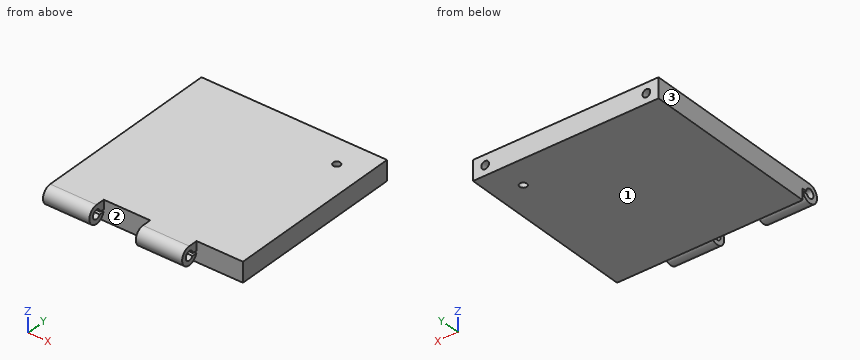
Autodesk Inventor part; units mm, degrees
ref_plane "YZ Plane" through (0, 0, 0) normal (1, 0, 0) x (0, 1, 0)
ref_plane "XZ Plane" through (0, 0, 0) normal (0, 1, 0) x (-1, 0, 0)
ref_plane "XY Plane" through (0, 0, 0) normal (0, 0, 1) x (1, 0, 0)
sketch "Sketch1" plane through (0, 0, 0) normal (0, 0, 1) x (1, 0, 0)
  line L0 (0, 0) -> (102.3, 0)
  line L1 (102.3, 0) -> (102.3, 100)
  line L2 (102.3, 100) -> (0, 100)
  line L3 (0, 100) -> (0, 0)
  dimension "d0" = 102.3
  dimension "d1" = 100
extrude "Extrusion1" add sketch "Sketch1" along normal blind 5
sketch "Sketch3" plane through (0, 0, 0) normal (-1, 0, 0) x (0, 0, 1)
  line L0 (5, 0) -> (0, 0)
  line L1 (0, 0) -> (0, -5)
  line L2 (0, -5) -> (5, -5)
  line L3 (5, -5) -> (5, 0)
  circle A0 centre (0, -5) radius 5
  circle A1 centre (0, -5) radius 2.5
  line L4 (-1.25, -2.8349) -> (-1.25, -0.1588)
  point P0 (0, 0)
  point P1 (0, -2.5)
  dimension "d15" = 5
  dimension "d16" = 5
  dimension "d17" = 5
  dimension "d18" = 2.5
  dimension "d19" = 1.25
extrude "Extrusion3" add sketch "Sketch3" against normal blind 25.575 contours L3 A0 L0 | A0 L2 A1 L1 | A0 L4 A1 L2
pattern_linear "Rectangular Pattern2" count 2 spacing 51.15 along (1, 0, 0) of "Extrusion3"
sketch "Sketch4" plane through (0, 0, 0) normal (0, 0, -1) x (-1, 0, 0)
  point P0 (0, 0)
sketch "Sketch5" plane through (0, 0, 0) normal (0, 0, -1) x (-1, 0, 0)
  line L0 (-102.3, 0) -> (-102.3, 100)
  line L1 (0, 0) -> (-102.3, 0)
  line L2 (-102.3, 0) -> (-102.3, 100)
  line L3 (-102.3, 100) -> (0, 100)
  line L4 (0, 100) -> (0, 0)
extrude "Extrusion4" add sketch "Sketch5" along normal blind 6
sketch "Sketch6" plane through (0, 0, 5) normal (0, 0, 1) x (1, 0, 0)
  line L0 (102.3, 100) -> (0, 100) construction
  line L1 (87.3, 100) -> (87.3, 84) construction
  line L2 (102.3, 0) -> (102.3, 100) construction
  point P0 (0, 0)
  dimension "d27" = 15
  dimension "d28" = 16
hole "Hole1" at (87.3, 84, 5) direction (0, 0, -1) diameter 4 end through all
sketch "Sketch8" plane through (51.15, -5, 5) normal (-1, 0, 0) x (0, 0, 1)
  point P0 (-5, 5)
sketch "Sketch9" plane through (0, 0, 5) normal (0, 0, 1) x (1, 0, 0)
  circle A0 centre (87.3, 84) radius 2 construction
  line L0 (87.3, 84) -> (102.3, 84) construction
  line L1 (102.3, 0) -> (102.3, 100) construction
  line L2 (87.3, 84) -> (87.3, 100) construction
  line L3 (76.725, 0) -> (102.3, 0)
  line L4 (102.3, 100) -> (0, 100)
  point P0 (0, 0)
  dimension "d45" = 15
  dimension "d46" = 16
  dimension "d57" = 100
sketch "Sketch10" plane through (0, 100, 5) normal (0, 1, 0) x (1, 0, 0)
  line L0 (0, 10) -> (0, 0) construction
  line L1 (0, 5.5) -> (102.7523, 5.5) construction
  line L2 (0, 11) -> (102.3, 11) construction
  point P0 (95.6, 5.5)
  point P1 (6.7, 5.5)
  point P2 (0, 6.25)
  dimension "d47" = 88.9
  dimension "d48" = 5.5
  dimension "d49" = 6.7
hole "Hole3" at (6.7, 100, -0.5) at (95.6, 100, -0.5) direction (0, -1, 0) diameter 4.25 depth 8 tip angle 118
properties part number "Hinge2"
The model under review builds one solid part; all positions refer to its coordinate system, in mm. Face numbers are marked on the shaded views. Give positions to 0.01 mm unless a question says otherwise; leave off trailing zeros. Loops run counter-clockwise (first coordinate to the right, second up) from the corner with the lowest first, then second, coordinate; pieces in that order, holes last. Notation, with made-up numbers: (-23, 17) -> (30, 17) arc R18 ccw to (30, 33) -> close; hole circle Ø8 at (-8, 35.25). An arc over 180 degrees is marked (long way). Answer as a JSON object with one key per item and string values. Group by question number.
Q1. Take a section at D-D (x = 31). Write out the cut boundary in (y, z), plus the area to 3 significant figures.
Q2. Take a section at C-C (x = 62.5). Write out the cut boundary in (y, z), plus the area to 3 significant figures.
Q3. Take a section at B-B (x = 87.3). Write out the cut boundary in (y, z).
Q4. Draft analysis for pull direction X (two halves, no side actions). For the marked faces 1, 2 and 3, state which applies: pulls with the +X half, pulls with the -X half, needs draft (parallel to the pull), parting line crosses it, or undercut.
Q5. Take a section at A-A (y = 84). Write out the cut boundary in (x, z).
Q6. Insertion check: pin 1 (2 mm diameter, centred on x = 18, y = -1.5, fed in from -Z); pin 2 (1 mm diameter, centred on x = 54.5, z = 3, fed in from -Y); pin 3 (1.5 mm diameter, centred on x = 47, z = 3, fed in from -Y). Each pin has a flat end and moves straight along its axis. Give the tip position at first contact, or say it passes through.
Q7. Wall thickness on line 1 along X through (y, z) = (84, -2.5); line 2 along Z through (x, y) = (6.7, 98.25) (3 decimals); line 3 along Z through (x, y) = (23, -5): over which ranges is each line inside the solid? List them lowest first.
Answer below:
{
 "1": {"outline": "(0, -6) -> (100, -6) -> (100, 5) -> (0, 5) -> close", "area": "1,100 mm2"},
 "2": {"outline": "(-5, 5) arc R5 ccw (long way) to (-0.16, -1.25) -> (-2.83, -1.25) arc R2.5 cw (long way) to (-2.5, 0) -> (0, 0) -> (0, -6) -> (100, -6) -> (100, 5) -> close", "area": "1,160 mm2"},
 "3": {"outline": "(0, -6) -> (82, -6) -> (82, 5) -> (0, 5) -> close; (86, -6) -> (100, -6) -> (100, 5) -> (86, 5) -> close"},
 "4": {"face 1": "needs draft", "face 2": "undercut", "face 3": "pulls with the -X half"},
 "5": {"outline": "(0, -6) -> (85.3, -6) -> (85.3, 5) -> (0, 5) -> close; (89.3, -6) -> (102.3, -6) -> (102.3, 5) -> (89.3, 5) -> close"},
 "6": {"pin 1": "stops at z = -4.33", "pin 2": "stops at y = -9.33", "pin 3": "stops at y = 0"},
 "7": {"line 1": "x = 0 to 85.3, 89.3 to 102.3", "line 2": "z = -6 to -2.625, 1.625 to 5", "line 3": "z = -5 to -2.5, 2.5 to 5"}
}
